Study the drawing (mm; zero at the part's minimum x, y, z) and answer. A direction names the side the tool comes from. Round coordinates to 2 decimals unless told otherwise and drop trailing zeros. Write each loop counter-clockwise with the first axis right and the second up, starting at its lowest first coordinate (ties: lowest second). Pieces come first, ordered by that corner, then holes. Notation, with made-up numbers: M 42.5,-9 L 99.5,-9 A19 ccw 99.5,-2 Z; hole C 8.5,-40 d8. An arc over 180 degrees is marked long. Write each question's results on one line, items separated by ' | '.
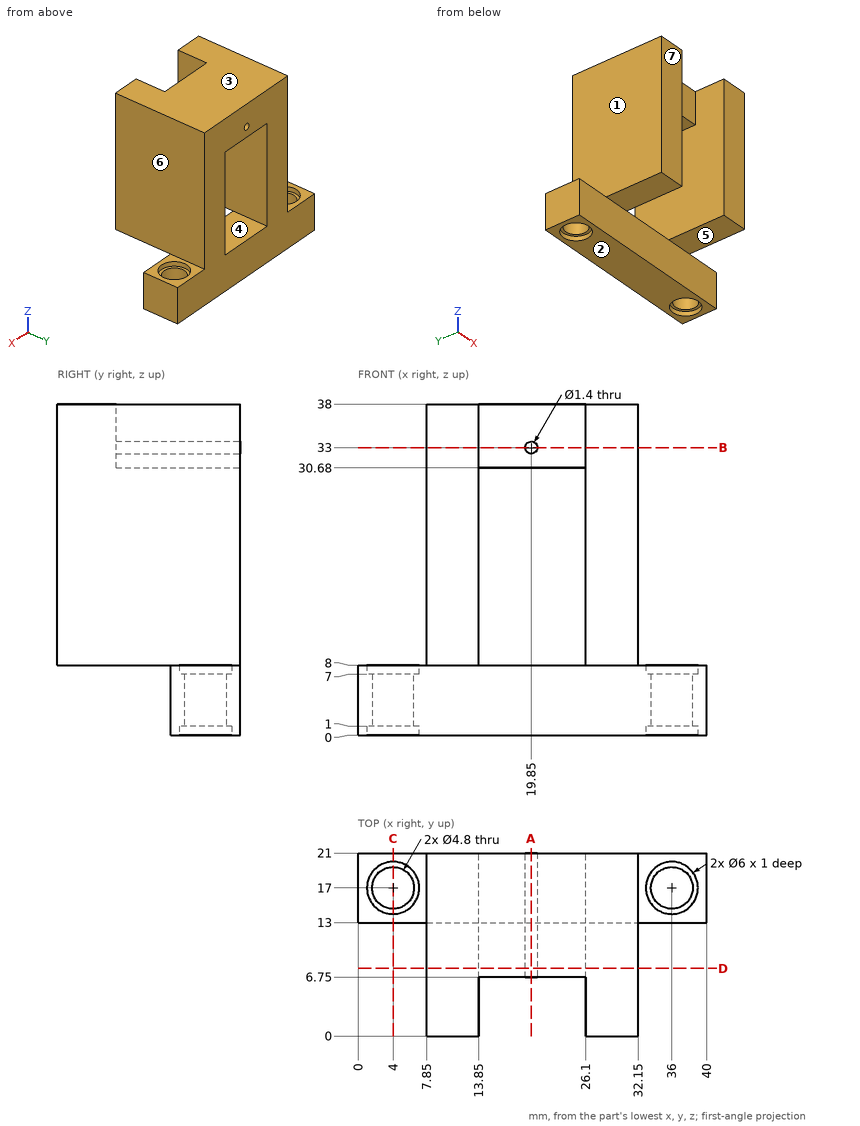
1) The mould has two halves that part along Z. Classify the marked faces 1, 2, 3 and 4: +Z half, -Z half, draft (parallel to the pull), parting line (faces both ways), or undercut.
Return value:
face 1: draft | face 2: -Z half | face 3: +Z half | face 4: undercut
2) Section A-A (x = 19.85) is taken. Determine the outline of the cut face in (y, z), then the cut area to 3 significant figures.
Return value:
outline: M 6.75,30.68 L 21,30.68 L 21,32.3 L 6.75,32.3 Z; M 6.75,33.7 L 21,33.7 L 21,38 L 6.75,38 Z; M 13,0 L 21,0 L 21,8 L 13,8 Z | area: 148 mm²
3) Section C-C (x = 4) is taken. Determine the outline of the cut face in (y, z), then the cut area to 3 significant figures.
Return value:
outline: M 13,0 L 14,0 L 14,1 L 14.6,1 L 14.6,7 L 14,7 L 14,8 L 13,8 Z; M 19.4,1 L 20,1 L 20,0 L 21,0 L 21,8 L 20,8 L 20,7 L 19.4,7 Z | area: 23.2 mm²
4) Section D-D (y = 7.75) is taken. Determine the outline of the cut face in (x, z), then the cut area to 3 significant figures.
Return value:
outline: M 7.85,8 L 13.85,8 L 13.85,30.68 L 26.1,30.68 L 26.1,8 L 32.15,8 L 32.15,38 L 7.85,38 Z; hole C 19.85,33 d1.4 | area: 450 mm²
5) Find the intervals of material crossed by line 1 (Z direction, x = 19.85, y = 14.5); line 2 (Y direction, x = 36, z = 4); line 3 (X direction, y = 3.25, z = 34), in increasing order.
Return value:
line 1: 0 to 8, 30.68 to 32.3, 33.7 to 38 | line 2: 13 to 14.6, 19.4 to 21 | line 3: 7.85 to 13.85, 26.1 to 32.15
6) A tool of negligible diameter and unlimited length cuts with its end or side. For the marked faces 5, 6 and 7, from which of +Z, -Z, +X, -X, +Y, -Y can it reach the whole face along a straight path? Write none if from no direction.
Return value:
face 5: -Z, +X, -X, -Y | face 6: +Z, +X, +Y, -Y | face 7: +Z, -Z, +X, -X, -Y
7) Section B-B (z = 33) is taken. Determine the outline of the cut face in (x, y).
Return value:
outline: M 7.85,0 L 13.85,0 L 13.85,6.75 L 19.15,6.75 L 19.15,21 L 7.85,21 Z; M 20.55,6.75 L 26.1,6.75 L 26.1,0 L 32.15,0 L 32.15,21 L 20.55,21 Z
8) Each of these flat-tipped pins is pushed along its axis until it touches: pin 1 (3.5 mm diameter, centred on x = 21, z = 34, fed in from -Y); pin 2 (10.5 mm diameter, centred on y = 7, z = 22, fed in from -X); pin 3 (7.5 mm diameter, centred on x = 36, y = 17, fed in from +Z); pin 4 (2 mm diameter, centred on x = 5.5, z = 18, fed in from +Y). Where does it stop, or does it pass through?
Return value:
pin 1: y = 6.75 | pin 2: x = 7.85 | pin 3: z = 8 | pin 4: through
